Design review of the part built by this model. Coordinates are the model's own, in mm. A direction names the side the tool comes from. Coordinates: 2 decimals unless noted, no trailing zeros.
Q1. For probe 1 along X at (y, z) = (50, -26); probe 2 along Z at (x, y) = (40, 2); probe 3 along Y at (x, z) = (14.5, 18.5), list the stretches that pass through material, from the lowest coordinate up.
Q2. Machinability: for faces 4 (the cylindrical face through (17.256, -47.247, -0.14)), 5 (the flat face through (17, 10.163, 56)), 6 (the cylindrical face through (54.11, 18.71, -9.26)), which of the approach directions +Z, -Z, +X, -X, +Y, -Y give a long, thin tool a straight path to every point of the face, cutting with its end or side? Answer none if there is none.
Q3. Insertion check: pin 1 (3 mm diameter, centred on x = 15.5, z = -3, fed in from +Y); pin 2 (1 mm diameter, centred on x = 32, y = -16, fed in from -Z); pin 3 (10 mm diameter, centred on y = 0, z = 50.419, fed in from +X). Each pin has a flat end and moves straight along its axis. Give the tip position at first contact, or say it passes through.
Q4. Mouldability with a two-part tool opening along X and no side actions: class faces 1 (the flat face through (44.45, -17, -10)), 2 (the conical face through (29.152, -11, -3.464)), 3 (the cylindrical face through (19.3, 39.02, 34.27)) as pulls with the +X half, pulls with the -X half, needs draft (parallel to the pull), parting line crosses it, or undercut.
Q5. Take a section at A-A (x = 25). State how many separate pieces and enclosed holes the cut face has, and give its area (3 significant figures).
```python
from build123d import *

# Parameters (mm, degrees)
HOUSING_2_DEPTH          = 44.45
SKETCH2_R                = 39.878
IMPELLER_CUT_DEPTH       = 22.4028
SKETCH4_R                = 9.641475923
INLET_CUT_DEPTH          = 19.8628
SKETCH6_R                = 3.175
FASTENER_BORE_DEPTH      = 116.84
FASTENER_PATTERN_COUNT   = 8
SKETCH7_R                = 100.114274451
SKETCH7_R_2              = 31.75
MASS_REDUCTION_CUT_DEPTH = 10.414
FILLET3_R                = 5.08
SKETCH8_W                = 34.036
SKETCH8_H                = 50.796537914
DISCHARGE_CUT_DEPTH      = 10.541
FILLET4_R                = 5.08
SKETCH9_R                = 2.54
DISCHARGE_BORE_DEPTH     = 50.038
SKETCH11_R               = 31.75
SKETCH11_R_2             = 9.641475923
BOSS_EXTRUDE1_DEPTH      = 19.05
SKETCH12_R               = 1.5875
CUT_EXTRUDE1_DEPTH       = 19.05
CIRPATTERN1_COUNT        = 6
FILLET6_R                = 5.08


with BuildPart() as part:
    # Sketch1 → Housing 2 (new body)
    with BuildSketch(Plane(origin=(0, 0, 0), x_dir=(0, 0, -1), z_dir=(1, 0, 0))):
        with BuildLine():
            Line((-60.96, 0), (-60.96, 60.96))
            Line((-60.96, 60.96), (0, 60.96))
            ThreePointArc((0, 60.96), (43.105229381, -43.105229381), (-60.96, 0))
        make_face()
    extrude(amount=HOUSING_2_DEPTH)

    # Sketch2 → Impeller Cut (cut)
    with BuildSketch(Plane.ZY):
        Circle(SKETCH2_R)
    extrude(amount=-IMPELLER_CUT_DEPTH, mode=Mode.SUBTRACT)

    # Sketch3 → Impeller Angle Cut (revolve, cut)
    with BuildSketch(Plane.XY, mode=Mode.PRIVATE) as impeller_angle_cut_sk:
        Polygon((29.602825054, 9.641475923), (22.4028, 39.878), (22.225, 0), (29.602825054, 0), align=None)
    revolve(impeller_angle_cut_sk.sketch.rotate(Axis((22.225, 0, 0), (1, 0, 0)), 180), axis=Axis((22.225, 0, 0), (1, 0, 0)), mode=Mode.SUBTRACT)

    # Sketch4 → Inlet Cut (cut)
    with BuildSketch(Plane.ZY.offset(-29.602825054)):
        with Locations(Location((0, 0, 0), (0, 0, 270))):
            Circle(SKETCH4_R)
    extrude(amount=-INLET_CUT_DEPTH, mode=Mode.SUBTRACT)

    # Sketch6 → Fastener Bore (cut)
    with BuildSketch(Plane(origin=(44.45, 0, 0), x_dir=(0, 0, -1), z_dir=(1, 0, 0))):
        with Locations((50.419, 0)):
            Circle(SKETCH6_R)
    fastener_bore = extrude(amount=-FASTENER_BORE_DEPTH, mode=Mode.SUBTRACT)

    # Fastener Pattern: Fastener Bore ×8 about axis, 1 skipped
    fastener_pattern_axis = Axis((0, 0, 0), (-1, 0, 0))
    add([fastener_bore.rotate(fastener_pattern_axis, i * 360 / FASTENER_PATTERN_COUNT) for i in range(1, FASTENER_PATTERN_COUNT) if i not in (5,)], mode=Mode.SUBTRACT)

    # Sketch7 → Mass Reduction Cut (cut)
    with BuildSketch(Plane(origin=(44.45, 0, 0), x_dir=(0, 0, -1), z_dir=(1, 0, 0))):
        Circle(SKETCH7_R)
        Circle(SKETCH7_R_2, mode=Mode.SUBTRACT)
    extrude(amount=-MASS_REDUCTION_CUT_DEPTH, mode=Mode.SUBTRACT)

    # Fillet3
    fillet3_edges = [part.edges().sort_by_distance(p)[0] for p in [
        (34.036, 0, 31.75),
    ]]
    fillet(fillet3_edges, radius=FILLET3_R)

    # Sketch8 → Discharge Cut (cut)
    with BuildSketch(Plane.XY.offset(60.96)):
        with Locations((17.018, 35.561731043)):
            Rectangle(SKETCH8_W, SKETCH8_H)
    extrude(amount=-DISCHARGE_CUT_DEPTH, mode=Mode.SUBTRACT)

    # Fillet4
    fillet4_edges = [part.edges().sort_by_distance(p)[0] for p in [
        (34.036, 5.081731043, 60.96),
        (34.036, -43.105229381, -43.105229381),
        (34.036, 60.96, 25.2095),
    ]]
    fillet(fillet4_edges, radius=FILLET4_R)

    # Sketch9 → Discharge Bore (cut)
    with BuildSketch(Plane.XY.offset(50.419)):
        with Locations((19.634252654, 36.501080952)):
            Circle(SKETCH9_R)
    extrude(amount=-DISCHARGE_BORE_DEPTH, mode=Mode.SUBTRACT)

    # Sketch11 → Boss-Extrude1 (add)
    with BuildSketch(Plane(origin=(44.45, 0, 0), x_dir=(0, 0, -1), z_dir=(1, 0, 0))):
        Circle(SKETCH11_R)
        with Locations(Location((0, 0, 0), (0, 0, 270))):
            Circle(SKETCH11_R_2, mode=Mode.SUBTRACT)
    extrude(amount=BOSS_EXTRUDE1_DEPTH)

    # Sketch12 → Cut-Extrude1 (cut)
    with BuildSketch(Plane(origin=(63.5, 0, 0), x_dir=(0, 0, -1), z_dir=(1, 0, 0))):
        with Locations((19.976045338, 0)):
            Circle(SKETCH12_R)
    cut_extrude1 = extrude(amount=-CUT_EXTRUDE1_DEPTH, mode=Mode.SUBTRACT)

    # CirPattern1: Cut-Extrude1 ×6 about axis
    cirpattern1_axis = Axis((0, 0, 0), (1, 0, 0))
    for i in range(1, CIRPATTERN1_COUNT):
        add(cut_extrude1.rotate(cirpattern1_axis, i * 360 / CIRPATTERN1_COUNT), mode=Mode.SUBTRACT)

    # Fillet6
    fillet6_edges = [part.edges().sort_by_distance(p)[0] for p in [
        (63.5, 0, 31.75),
    ]]
    fillet(fillet6_edges, radius=FILLET6_R)


solid = part.part
```
Response:
1. probe 1: x = 0 to 34.01
1. probe 2: z = -31.69 to -9.43, 9.43 to 31.69
1. probe 3: y = -58.09 to -35.33, 35.33 to 60.96
2. face 4: +X, -X
2. face 5: +Z, +X, -X, +Y
2. face 6: +X
3. pin 1: stops at y = 60.94
3. pin 2: stops at z = -58.14
3. pin 3: stops at x = 34.04
4. face 1: pulls with the +X half
4. face 2: pulls with the -X half
4. face 3: undercut
5. separate pieces: 1
5. enclosed holes: 8
5. area: 9,080 mm2
